```python
from build123d import *

# Parameters (mm, degrees)
SKETCH1_R           = 1.905
SKETCH1_R_2         = 3.175
BOSS_EXTRUDE1_DEPTH = 2.54


with BuildPart() as part:
    # Sketch1 → Boss-Extrude1 (new body)
    with BuildSketch(Plane(origin=(0, 0, 0), x_dir=(1, 0, 0), z_dir=(0, 1, 0))):
        with BuildLine():
            Line((12.7, -76.2), (12.7, -14.199031657))
            ThreePointArc((12.7, -14.199031657), (0, 19.05), (-12.7, -14.199031657))
            Line((-12.7, -14.199031657), (-12.7, -76.2))
            Line((-12.7, -76.2), (12.7, -76.2))
        make_face()
        with Locations((9.525, 0)):
            Circle(SKETCH1_R, mode=Mode.SUBTRACT)
        with Locations((-9.525, 0)):
            Circle(SKETCH1_R, mode=Mode.SUBTRACT)
        with Locations((0, 7.9375)):
            Circle(SKETCH1_R, mode=Mode.SUBTRACT)
        with Locations((0, -7.9375)):
            Circle(SKETCH1_R, mode=Mode.SUBTRACT)
        Circle(SKETCH1_R_2, mode=Mode.SUBTRACT)
    extrude(amount=BOSS_EXTRUDE1_DEPTH)


solid = part.part
```
Verification items for the finished model (mm, model axes). A direction names the side the tool comes from. Round coordinates to 2 decimals unless told otherwise and drop trailing zeros. Write each loop counter-clockwise with the first axis right and the second up, starting at its lowest first coordinate (ties: lowest second). Pieces come first, ordered by that corner, then holes.
1. Draft check along X on faces 1 (the cylindrical face through (-0.248, 1.252, -9.826)), 2 (the cylindrical face through (0.64, 1.25, -19.04)), 3 (the flat face through (0, 1, 76.2)). Enter one of: +X half, -X half, draft (parallel to the pull), parting line (faces both ways), or undercut.
2. Scan lines: L1, parallel to X at y = 1.85, z = 0 (3 decimals); L2, parallel to X at y = 1.9, z = 39; L3, parallel to X at y = 1.2, z = -8.5. Record each from-to range of solid material in increasing order.
3. Section check C-C on x = 10. Enter the section's corners in (y, z).
4. Access from +Z, -Z, +X, -X, +Y, -Y to the whole of each face (thin tool, end or side, straight path). Record for faces 4 (the flat face through (0, 2.54, 28)), 5 (the flat face through (12.7, 1, 46)), 6 (the flat face through (-12.7, 1, 45)).
5. Section check B-B on z = 0. Enter the section's corners in (x, y) (3 decimals), plus the area to 3 significant figures.
6. Section check A-A on x = 0. State how many separate pieces and enclosed holes the cut face has, plus the area to 3 significant figures.
7. Gauge pin test, flat ends, axial feed: P1, Ø0.8, axis at y = 1.5, z = 36.5, coming from the -X side; P2, Ø0.8, axis at y = 1, z = 47, coming from the +X side; P3, Ø4, axis at x = 0, z = 0, coming from the -Y side; P4, Ø1, axis at x = 14.5, y = 2, coming from the -Z side. Record the tip position at first contact, or that the pin passes through.
Answer:
1. face 1: undercut
1. face 2: parting line
1. face 3: draft
2. L1: x = -19.05 to -11.43, -7.62 to -3.175, 3.175 to 7.62, 11.43 to 19.05
2. L2: x = -12.7 to 12.7
2. L3: x = -17.05 to -1.82, 1.82 to 17.05
3. outline: (0, -16.21) - (2.54, -16.21) - (2.54, -1.84) - (0, -1.84) - close; (0, 1.84) - (2.54, 1.84) - (2.54, 76.2) - (0, 76.2) - close
4. face 4: +Z, -Z, +X, -X, +Y
4. face 5: +Z, +X, +Y, -Y
4. face 6: +Z, -X, +Y, -Y
5. outline: (-19.05, 0) - (-11.43, 0) - (-11.43, 2.54) - (-19.05, 2.54) - close; (-7.62, 0) - (-3.175, 0) - (-3.175, 2.54) - (-7.62, 2.54) - close; (3.175, 0) - (7.62, 0) - (7.62, 2.54) - (3.175, 2.54) - close; (11.43, 0) - (19.05, 0) - (19.05, 2.54) - (11.43, 2.54) - close
5. area: 61.3 mm2
6. separate pieces: 4
6. enclosed holes: 0
6. area: 206 mm2
7. P1: stops at x = -12.7
7. P2: stops at x = 12.7
7. P3: passes through
7. P4: stops at z = -12.92
